```python
from build123d import *

# Parameters (mm, degrees)
F0_R     = 10.85
F1_DEPTH = 7


with BuildPart() as f1:
    # F0 (on Top) → F1 (new body)
    with BuildSketch(Plane.XY):
        with BuildLine():
            Line((-17.5, -10.10363), (-9.862379, -14.513212))
            Line((-9.862379, -14.513212), (-9.862379, -47.222504))
            ThreePointArc((-9.862379, -47.222504), (-20.463736, -64.844891), (0.071775, -65.953967))
            ThreePointArc((0.071775, -65.953967), (20.833211, -65.236064), (9.862379, -47.595388))
            Line((9.862379, -47.595388), (9.862379, -14.513212))
            Line((9.862379, -14.513212), (17.5, -10.10363))
            Line((17.5, -10.10363), (17.5, -1.284465))
            Line((17.5, -1.284465), (45.827078, 15.070181))
            ThreePointArc((45.827078, 15.070181), (66.389191, 14.70033), (57.081923, 33.039142))
            ThreePointArc((57.081923, 33.039142), (46.079483, 50.660122), (36.287625, 32.338765))
            Line((36.287625, 32.338765), (7.637621, 15.797677))
            Line((7.637621, 15.797677), (0, 20.207259))
            Line((0, 20.207259), (-7.637621, 15.797677))
            Line((-7.637621, 15.797677), (-35.964699, 32.152323))
            ThreePointArc((-35.964699, 32.152323), (-45.925454, 50.144561), (-57.153698, 32.914825))
            ThreePointArc((-57.153698, 32.914825), (-66.912694, 14.575942), (-46.150004, 15.256623))
            Line((-46.150004, 15.256623), (-17.5, -1.284465))
            Line((-17.5, -1.284465), (-17.5, -10.10363))
        make_face()
        Circle(F0_R, mode=Mode.SUBTRACT)
    extrude(amount=F1_DEPTH)


solid = f1.part
```
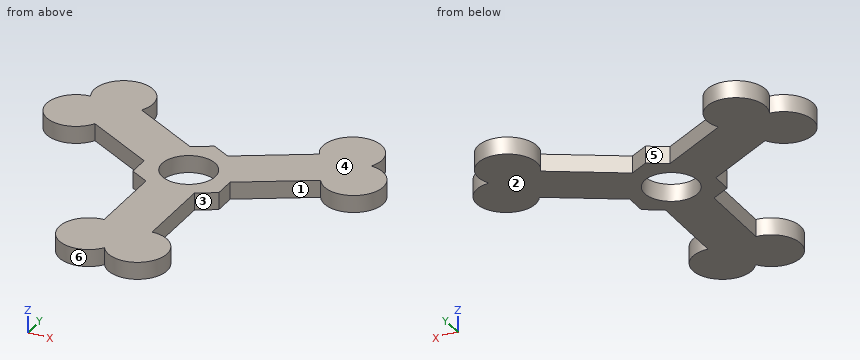
CAD build for the part. Positions are in the model's coordinates, mm. Face numbers are marked on the shaded views. A direction names the side the tool comes from. Give positions to 0.01 mm unless a question says otherwise; leave off trailing zeros. Write each loop counter-clockwise with the first axis right and the second up, starting at its lowest first coordinate (ties: lowest second). Pieces come first, ordered by that corner, then holes. Notation, with made-up numbers: (7.25, -35.75) -> (54.25, -35.75) arc R11 cw to (54.25, -29.75) -> close; hole circle Ø11 at (39, -26.75). An arc over 180 degrees is marked (long way). Write each question's results on one line, items separated by ' | '.
1. Two-plate mould, pull along Y, no slides. Class the marked faces 4, 5 and 6: pulls with the +Y half, pulls with the -Y half, needs draft (parallel to the pull), parting line crosses it, or undercut.
Geometry check:
face 4: needs draft | face 5: pulls with the +Y half | face 6: undercut
2. Drop flat-ended pins along their axis: P1, Ø12, axis at x = -22, y = 25, coming from the -Z side; P2, Ø3.5, axis at y = -32.5, z = 4.5, coming from the -X side; P3, Ø3.5, axis at y = -26, z = 3, coming from the +X side; P4, Ø3, axis at y = 0.5, z = 3, coming from the +X side. Give the stop position or say it passes through.
Geometry check:
P1: z = 0 | P2: x = -9.86 | P3: x = 9.86 | P4: x = 23.19
3. Cut at A-A, the plane x = -12.5. Write the cut outline in (y, z).
Geometry check:
outline: (-70.93, 0) -> (-47.52, 0) -> (-47.52, 7) -> (-70.93, 7) -> close; (-12.99, 0) -> (18.6, 0) -> (18.6, 7) -> (-12.99, 7) -> close
4. Cut at C-C, the plane y = -6. Write the cut outline in (x, z), then the cut area to 3 significant figures.
Geometry check:
outline: (-17.5, 0) -> (-9.04, 0) -> (-9.04, 7) -> (-17.5, 7) -> close; (9.04, 0) -> (17.5, 0) -> (17.5, 7) -> (9.04, 7) -> close | area: 118 mm²
5. Wall check: probe 1 along X at (y, z) = (-24, 4); probe 2 along Y at (x, z) = (-13, 5); probe 3 along X at (y, z) = (-1.5, 5.75). Give the ranges that are in metal, low to high. Write a range as [from, to].
Geometry check:
probe 1: [-9.86, 9.86] | probe 2: [-70.81, -47.64], [-12.7, 18.89] | probe 3: [-17.5, -10.75], [10.75, 17.5]
6. Which spindle directions (+Z, -Z, +X, -X, +Y, -Y) get a long thin tool onto all of the face, cutting with end or side? Do the marked faces 1, 2 and 3. Say none if no direction does.
Geometry check:
face 1: +Z, -Z | face 2: -Z, +X, -X, +Y, -Y | face 3: +Z, -Z, +X
7. Cut at D-D, the plane x = 41. Write the cut outline in (y, z).
Geometry check:
outline: (12.28, 0) -> (49.34, 0) -> (49.34, 7) -> (12.28, 7) -> close
8. Cut at B-B, the plane z = 3.75. Write the cut outline in (x, y).
Geometry check:
outline: (-57.15, 32.91) arc R12 ccw (long way) to (-46.15, 15.26) -> (-17.5, -1.28) -> (-17.5, -10.1) -> (-9.86, -14.51) -> (-9.86, -47.22) arc R12 ccw (long way) to (0.07, -65.95) arc R12 ccw (long way) to (9.86, -47.6) -> (9.86, -14.51) -> (17.5, -10.1) -> (17.5, -1.28) -> (45.83, 15.07) arc R12 ccw (long way) to (57.08, 33.04) arc R12 ccw (long way) to (36.29, 32.34) -> (7.64, 15.8) -> (0, 20.21) -> (-7.64, 15.8) -> (-35.96, 32.15) arc R12 ccw (long way) to start; hole circle Ø21.7 at (0, 0)
